from build123d import *

# Parameters (mm, degrees)
SKETCH_1_R          = 2.2
EXTRUDE_1_DEPTH     = 2.4
EXTRUDE_START       = 2.4
SKETCH_1_4_R        = 1.15
EXTRUDE_2_DEPTH     = 54.8
CUT_EXTRUDE_1_DEPTH = 1.5


with BuildPart() as part:
    # 草图1 → 凸台-拉伸1 (new body)
    with BuildSketch(Plane(origin=(0, 0, 0), x_dir=(1, 0, 0), z_dir=(0, 1, 0))):
        with Locations(Location((0, 0, 0), (0, 0, 270))):
            Circle(SKETCH_1_R)
    extrude(amount=EXTRUDE_1_DEPTH)

    # 草图1<4> → 凸台-拉伸2 (add)
    with BuildSketch(Plane(origin=(0, 0, 0), x_dir=(1, 0, 0), z_dir=(0, 1, 0)).offset(EXTRUDE_START)):
        with Locations(Location((0, 0, 0), (0, 0, 90))):
            Circle(SKETCH_1_4_R)
    extrude(amount=EXTRUDE_2_DEPTH)

    # 草图1<3> → 切除-拉伸1 (cut)
    with BuildSketch(Plane(origin=(0, 0, 0), x_dir=(1, 0, 0), z_dir=(0, 1, 0))):
        with BuildLine():
            ThreePointArc((1.15, 0), (1.149992705, 0.004096081), (1.149970821, 0.008192111))
            Line((1.149970821, 0.008192111), (0.582079986, 0.991807889))
            ThreePointArc((0.582079986, 0.991807889), (0.575, 0.995929214), (0.567890835, 1))
            Line((0.567890835, 1), (-0.567890835, 1))
            ThreePointArc((-0.567890835, 1), (-0.575, 0.995929214), (-0.582079986, 0.991807889))
            Line((-0.582079986, 0.991807889), (-1.149970821, 0.008192111))
            ThreePointArc((-1.149970821, 0.008192111), (-1.15, 0), (-1.149970821, -0.008192111))
            Line((-1.149970821, -0.008192111), (-0.582079986, -0.991807889))
            ThreePointArc((-0.582079986, -0.991807889), (-0.575, -0.995929214), (-0.567890835, -1))
            Line((-0.567890835, -1), (0.567890835, -1))
            ThreePointArc((0.567890835, -1), (0.575, -0.995929214), (0.582079986, -0.991807889))
            Line((0.582079986, -0.991807889), (1.149970821, -0.008192111))
            ThreePointArc((1.149970821, -0.008192111), (1.149992705, -0.004096081), (1.15, 0))
        make_face()
    extrude(amount=CUT_EXTRUDE_1_DEPTH, mode=Mode.SUBTRACT)


solid = part.part
Read the model definition and answer for the solid it produces. Units are mm, in the model's axes. A direction names the side the tool comes from. Give positions to 0.01 mm unless a question says otherwise; leave off trailing zeros. Write each loop counter-clockwise with the first axis right and the second up, starting at its lowest first coordinate (ties: lowest second). Pieces come first, ordered by that corner, then holes. Notation, with made-up numbers: (83, 25) - (120, 25) arc R23 ccw to (120, 38) - close; hole circle Ø2 at (-5.5, 44.25). An arc over 180 degrees is marked (long way). Answer in a Markdown table with one row per item. Add a question column.
Item 1: Flat-ended cylindrical pins translate along their axes: P1, Ø1.5, axis at x = -1, y = 46.5, coming from the -Z side; P2, Ø1.5, axis at x = -1.5, y = 25.5, coming from the +Z side; P3, Ø2, axis at y = 38.5, z = -1.5, coming from the +X side. Find the tip coordinate at first contact, or state that the pin passes through.
Item 2: Section A-A, the plane x = 0 is taken. Write down the section's boundary in (y, z), and give its area (3 significant figures).
Item 3: Find the intervals of material crossed by L1, parallel to Y at x = -1.3, z = 0.9; L2, parallel to Z at x = -1, y = 26; L3, parallel to Y at x = -1, z = 0, in increasing order.
Item 4: Determine the mould class of faces 4 (the face through (-1, 2.4, 1)), 5 (the face through (0, 1.5, 0)), 6 (the face through (2.18, 1.18, -0.29)) for opening direction X: pulls with the +X half, pulls with the -X half, needs draft (parallel to the pull), parting line crosses it, or undercut.
Item 5: A tool of negligible diameter and unlimited length cuts with its end or side. For faces 1 (the face through (-0.345, 29.416, -1.097)), 2 (the face through (0, 57.2, 0)), 3 (the face through (-0.87, 0.74, 0.49)), from which of +Z, -Z, +X, -X, +Y, -Y can it reach the whole face along a straight path? Write none if from no direction.
Item 6: Section B-B, the plane y = 27 is taken. Write down the section's boundary in (x, z), and give its area (3 significant figures).
Recorded:
| question | item | result |
|---|---|---|
| 1 | P1 | stops at z = -1.12 |
| 1 | P2 | stops at z = 0.87 |
| 1 | P3 | stops at x = 1.04 |
| 2 | outline | (0, -2.2) - (2.4, -2.2) - (2.4, -1.15) - (57.2, -1.15) - (57.2, 1.15) - (2.4, 1.15) - (2.4, 2.2) - (0, 2.2) - (0, 1) - (1.5, 1) - (1.5, -1) - (0, -1) - close |
| 2 | area | 134 mm2 |
| 3 | L1 | y = 0 to 2.4 |
| 3 | L2 | z = -0.57 to 0.57 |
| 3 | L3 | y = 1.5 to 57.2 |
| 4 | face 4 | needs draft |
| 4 | face 5 | undercut |
| 4 | face 6 | parting line crosses it |
| 5 | face 1 | +Y |
| 5 | face 2 | +Z, -Z, +X, -X, +Y |
| 5 | face 3 | -Y |
| 6 | outline | circle Ø2.3 at (0, 0) |
| 6 | area | 4.15 mm2 |
